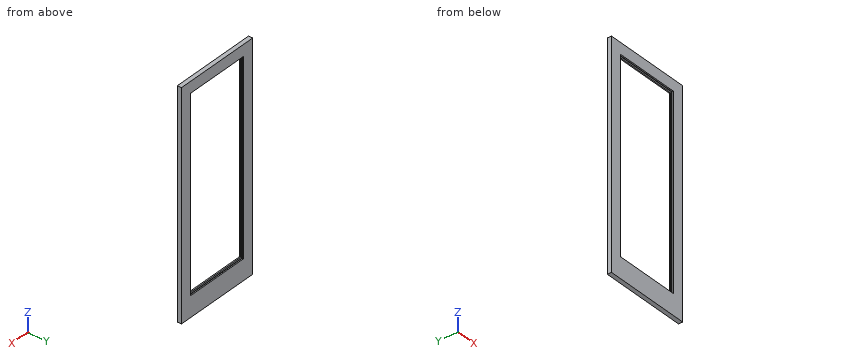
```python
from build123d import *

# Parameters (mm, degrees)
F0_W     = 918
F0_H     = 2370
F0_W_2   = 678
F0_H_2   = 2030
F1_DEPTH = 44
F2_W     = 708
F2_H     = 2060
F2_W_2   = 678
F2_H_2   = 2030
F3_DEPTH = 31
F4_W     = 708
F4_H     = 2060
F4_W_2   = 678
F4_H_2   = 2030
F5_DEPTH = 12


with BuildPart() as f1:
    # F0 (on Front) → F1 (new body)
    with BuildSketch(Plane.XZ):
        with Locations((-459, 1185)):
            Rectangle(F0_W, F0_H)
        with Locations((-459, 1235)):
            Rectangle(F0_W_2, F0_H_2, mode=Mode.SUBTRACT)
    extrude(amount=F1_DEPTH)

    # F2 (on face) → F3 (cut)
    with BuildSketch(Plane(origin=(0, 0, 0), x_dir=(-1, 0, 0), z_dir=(0, 1, 0))):
        with Locations((459, 1235)):
            Rectangle(F2_W, F2_H)
        with Locations((459, 1235)):
            Rectangle(F2_W_2, F2_H_2, mode=Mode.SUBTRACT)
    extrude(amount=-F3_DEPTH, mode=Mode.SUBTRACT)

    # F4 (on face) → F5 (join)
    with BuildSketch(Plane(origin=(0, 0, 0), x_dir=(-1, 0, 0), z_dir=(0, 1, 0))):
        with Locations((459, 1235)):
            Rectangle(F4_W, F4_H)
        with Locations((459, 1235)):
            Rectangle(F4_W_2, F4_H_2, mode=Mode.SUBTRACT)
    extrude(amount=-F5_DEPTH)


solid = f1.part
```
Check sheet for the modelled part. Datum: model origin and axes. Units: mm. Coordinates: 2 decimals unless noted, no trailing zeros. Order: outer loops, then holes, each group sorted by start corner. A loop starts at its lowest first (then second) coordinate and runs counter-clockwise, first axis right, second up. Notation, with made-up numbers: (37.25, -28) -> (77.25, -28) arc R29 ccw to (77.25, 8) -> close; hole circle Ø7 at (-38, 84). An arc over 180 degrees is marked (long way). Write item = value, one per line. Start each with the question number.
1) Cross-section at A-A (x = -591). Enter the section's corners in (y, z).
2) Cross-section at B-B (y = -21.5). Enter the section's corners in (x, z), then the cut area to 3 significant figures.
3) Cross-section at C-C (z = 1198). Enter the section's corners in (x, y).
4) Material ranges on L1, parallel to Z at x = -334.5, y = -13.5; L2, parallel to X at y = -39.5, z = 699; L3, parallel to Z at x = -773, y = -37.5, recorded low to high.
Ans:
q1.outline = (-44, 0) -> (0, 0) -> (0, 220) -> (-12, 220) -> (-12, 205) -> (-31, 205) -> (-31, 220) -> (-44, 220) -> close; (-44, 2250) -> (-31, 2250) -> (-31, 2265) -> (-12, 2265) -> (-12, 2250) -> (0, 2250) -> (0, 2370) -> (-44, 2370) -> close
q2.outline = (-918, 0) -> (0, 0) -> (0, 2370) -> (-918, 2370) -> close; hole (-813, 205) -> (-105, 205) -> (-105, 2265) -> (-813, 2265) -> close
q2.area = 717,000 mm²
q3.outline = (-918, -44) -> (-798, -44) -> (-798, -31) -> (-813, -31) -> (-813, -12) -> (-798, -12) -> (-798, 0) -> (-918, 0) -> close; (-120, -44) -> (0, -44) -> (0, 0) -> (-120, 0) -> (-120, -12) -> (-105, -12) -> (-105, -31) -> (-120, -31) -> close
q4.L1 = 0 to 205, 2265 to 2370
q4.L2 = -918 to -798, -120 to 0
q4.L3 = 0 to 220, 2250 to 2370
